from build123d import *

# Parameters (mm, degrees)
BOSS_EXTRUDE1_DEPTH = 9
SKETCH4_R           = 11.5
SKETCH4_R_2         = 1.5
CUT_EXTRUDE1_DEPTH  = 80.001582263
SKETCH5_W           = 9
SKETCH5_H           = 25
CUT_EXTRUDE2_DEPTH  = 80.001582263
SKETCH6_W           = 15
SKETCH6_H           = 9
CUT_EXTRUDE3_DEPTH  = 80.001582263


with BuildPart() as part:
    # Sketch2 → Boss-Extrude1 (new body)
    with BuildSketch(Plane(origin=(0, 0, 0), x_dir=(1, 0, 0), z_dir=(0, 1, 0))):
        Polygon((-50, 46.5), (-50, -46.5), (-35, -46.5), (-35, -37.5), (-15, -37.5), (-15, -46.5), (15, -46.5), (15, -37.5), (35, -37.5), (35, -46.5), (50, -46.5), (50, 46.5), (35, 46.5), (35, 37.5), (15, 37.5), (15, 60.5), (-15, 60.5), (-15, 37.5), (-35, 37.5), (-35, 46.5), align=None)
    extrude(amount=BOSS_EXTRUDE1_DEPTH)

    # Sketch4 → Cut-Extrude1 (cut, through all)
    with BuildSketch(Plane(origin=(0, 9, 0), x_dir=(1, 0, 0), z_dir=(0, 1, 0))):
        with Locations(Location((0, 17.5, 0), (0, 0, 270))):
            Circle(SKETCH4_R)
        with Locations(Location((-15.5, 2, 0), (0, 0, 270))):
            Circle(SKETCH4_R_2)
        with Locations(Location((15.5, 2, 0), (0, 0, 90))):
            Circle(SKETCH4_R_2)
        with Locations(Location((15.5, 33, 0), (0, 0, 270))):
            Circle(SKETCH4_R_2)
        with Locations(Location((-15.5, 33, 0), (0, 0, 90))):
            Circle(SKETCH4_R_2)
    extrude(amount=-CUT_EXTRUDE1_DEPTH, mode=Mode.SUBTRACT)

    # Sketch5 → Cut-Extrude2 (cut, through all)
    with BuildSketch(Plane(origin=(0, 9, 0), x_dir=(1, 0, 0), z_dir=(0, 1, 0))):
        with Locations((-45.5, 0)):
            Rectangle(SKETCH5_W, SKETCH5_H)
        with Locations((45.5, 0)):
            Rectangle(SKETCH5_W, SKETCH5_H)
    extrude(amount=-CUT_EXTRUDE2_DEPTH, mode=Mode.SUBTRACT)

    # Sketch6 → Cut-Extrude3 (cut, through all)
    with BuildSketch(Plane(origin=(0, 9, 0), x_dir=(1, 0, 0), z_dir=(0, 1, 0))):
        with Locations((-42.5, 42)):
            Rectangle(SKETCH6_W, SKETCH6_H)
        with Locations((42.5, 42)):
            Rectangle(SKETCH6_W, SKETCH6_H)
    extrude(amount=-CUT_EXTRUDE3_DEPTH, mode=Mode.SUBTRACT)


solid = part.part
Design review of the part built by this model. Coordinates are the model's own, in mm. A direction names the side the tool comes from. Coordinates: 2 decimals unless noted, no trailing zeros. Order: outer loops, then holes, each group sorted by start corner. A loop starts at its lowest first (then second) coordinate and runs counter-clockwise, first axis right, second up.
Item 1: For line 1 (X direction, y = 5, z = -2); line 2 (Z direction, x = 16.5, y = 3); line 3 (X direction, y = 3.5, z = -33), list the stretches that pass through material, from the lowest coordinate up.
Item 2: Take a section at B-B, the plane x = 0. Write out the cut boundary in (y, z).
Item 3: Take a section at A-A, the plane z = -2. Write out the cut boundary in (x, y).
Item 4: For pin 1 Ø2.5 at (x, y) = (-27.5, 5) entering from -Z; pin 2 Ø3.5 at (x, z) = (-15.5, -2) entering from +Y; pin 3 Ø4.5 at (y, z) = (6, -51.5) entering from -X; pin 4 Ø4.5 at (y, z) = (5.5, -51) entering from +X, all flat-tipped, find the tip position at first contact; note any pin that passes through.
Item 5: For faces 1 (the flat face through (45, 5, 12.5)), 2 (the flat face through (-15, 4, -49)), 3 (the flat face through (-46, 5, -12.5)), 4 (the flat face through (15, 4, -49)), 5 (the flat face through (35, 4, 42)), list the 3-axis set-ups (+Z, -Z, +X, -X, +Y, -Y) from which the entire face can be reached by the end or side of a thin tool; tool diameter is ignored.
Item 6: Take a section at D-D, the plane y = 3. Count the separate pieces of the cut face and the enclosed holes in it, then the cut area to 3 significant figures.
Item 7: The part is to be moulded in two halves that separate along X. For faces 6 (the flat face through (-50, 4, -25)), 7 (the flat face through (0, 4, 46.5)), 8 (the cylindrical face through (14.6, 4.6, -34.2)), say which applies: pulls with the +X half, pulls with the -X half, needs draft (parallel to the pull), parting line crosses it, or undercut.
Item 8: Take a section at C-C, the plane z = -17.5. Write out the cut boundary in (x, y).
The answers:
1. line 1: x = -41 to -17, -14 to 14, 17 to 41
1. line 2: z = -37.5 to -34.12, -31.88 to -3.12, -0.88 to 37.5
1. line 3: x = -50 to -17, -14 to 14, 17 to 50
2. outline: (0, -60.5) - (9, -60.5) - (9, -29) - (0, -29) - close; (0, -6) - (9, -6) - (9, 46.5) - (0, 46.5) - close
3. outline: (-41, 0) - (-17, 0) - (-17, 9) - (-41, 9) - close; (-14, 0) - (14, 0) - (14, 9) - (-14, 9) - close; (17, 0) - (41, 0) - (41, 9) - (17, 9) - close
4. pin 1: stops at z = -37.5
4. pin 2: stops at y = 9
4. pin 3: stops at x = -15
4. pin 4: stops at x = 15
5. face 1: +X, +Y, -Y
5. face 2: -Z, -X, +Y, -Y
5. face 3: -X, +Y, -Y
5. face 4: -Z, +X, +Y, -Y
5. face 5: +Z, +Y, -Y
6. separate pieces: 1
6. enclosed holes: 5
6. area: 7,840 mm2
7. face 6: pulls with the -X half
7. face 7: needs draft
7. face 8: undercut
8. outline: (-50, 0) - (-11.5, 0) - (-11.5, 9) - (-50, 9) - close; (11.5, 0) - (50, 0) - (50, 9) - (11.5, 9) - close
